Source: CAD feature listing. Evaluate the final solid. Frame: model axes, mm. A direction names the side the tool comes from. Coordinates: 2 decimals unless noted, no trailing zeros. Order: outer loops, then holes, each group sorted by start corner. A loop starts at its lowest first (then second) coordinate and runs counter-clockwise, first axis right, second up. Notation, with made-up numbers: (-25.75, -17) -> (24.25, -17) arc R23 ccw to (24.25, 0) -> close; hole circle Ø11 at (-21, 86.25). An arc over 180 degrees is marked (long way). Write each question's results on one line, items separated by ' | '. Start each with the question number.
Autodesk Inventor part; units mm, degrees
ref_plane "WorkPlane1" through (0, 0, 0) normal (0, 0, 1) x (1, 0, 0)
ref_plane "MSC_PF1" through (0, 0, 0) normal (1, 0, 0) x (0, 1, 0)
ref_plane "MSC_PT1" through (0, 0, 0) normal (0, 0, -1) x (-1, 0, 0)
ref_plane "WorkPlane1" through (0, 0, 0) normal (0, 0, 1) x (1, 0, 0)
sketch "Sketch1" plane through (0, 0, 0) normal (0, 0, 1) x (1, 0, 0)
  point P0 (0, 0)
sketch "Sketch2" plane through (0, 0, 0) normal (0, 0, 1) x (1, 0, 0)
  line L0 (-6.5, 3.7529) -> (-6.5, -3.7529)
  line L1 (0, 7.5054) -> (-6.5, 3.7529)
  line L2 (6.5, 3.7529) -> (0, 7.5054)
  line L3 (6.5, -3.7529) -> (6.5, 3.7529)
  line L4 (0, -7.5054) -> (6.5, -3.7529)
  line L5 (-6.5, -3.7529) -> (0, -7.5054)
  circle A0 centre (0, 0) radius 6.5 construction
  dimension "d1" = 13
  dimension "d29" = 0
  dimension "d30" = 0
extrude "Extrusion1" add sketch "Sketch2" along normal blind 5.3
sketch "Sketch3" plane through (0, 0, 0) normal (1, 0, 0) x (0, 1, 0)
  line L0 (6.5, 5.3) -> (7.6054, 5.3)
  line L1 (7.6054, 4.6618) -> (6.5, 5.3)
  line L2 (7.6054, 5.3) -> (7.6054, 4.6618)
  line L3 (0, -1.06) -> (0, 6.36)
  line L4 (7.5054, 0) -> (7.5054, 5.3)
  dimension "d25" = 0.1
  dimension "d26" = 0
  dimension "d27" = 60
  dimension "d28" = 6.5
revolve "Revolution1" cut sketch "Sketch3" angle 360 about axis through (0, 0, -10) along (0, 0, 1)
sketch "Sketch4" plane through (0, 0, 0) normal (1, 0, 0) x (0, 1, 0)
  line L0 (0, -30) -> (0, 0)
  line L1 (-4, -30) -> (0, -30)
  line L2 (-4, 0) -> (-4, -30)
  line L3 (0, 0) -> (-4, 0)
  line L4 (0, -30) -> (0, 0)
  line L5 (-4.8, 0) -> (0.8, 0)
  line L6 (0, -36) -> (0, 6)
  dimension "d18" = 4
  dimension "d20" = 30
  dimension "d33" = 0
  dimension "d34" = 0
revolve "Revolution2" add sketch "Sketch4" angle 360 about axis through (0, 0, -30) along (0, 0, -1)
chamfer "Chamfer1" distance 0.625 angle 45 1 edges at (0, 4, -30)
fillet "Fillet1" radius 0.4 1 edges at (0, 4, 0)
thread "Thread1"
ref_plane "MSC_PF1" through (0, 0, 0) normal (1, 0, 0) x (0, 1, 0)
ref_plane "MSC_PT1" through (0, 0, 0) normal (0, 0, -1) x (-1, 0, 0)
equation "\"d22\" = 0.5 * PTC"
equation "\"d23\" = 0.5 * PTC"
equation "\"d24\" = r"
equation "\"d1\" = ParS"
equation "\"d6\" = ParK"
equation "\"b\" = NLG - 2 * PTC"
equation "\"d28\" = 0.5 * ParS"
equation "\"d18\" = 0.5 * NND"
equation "\"d20\" = NLG"
equation "\"NND\" = 8"
equation "\"NLG\" = 30"
equation "\"PTC\" = 1.25"
equation "\"ParK\" = 5.3"
equation "\"ParS\" = 13"
equation "\"msp_es\" = 0.577367 * ParS"
equation "\"r\" = 0.4"
equation "\"THREADDIA\" = NND"
properties part number "ISO 4018 - M8 x 30" material "Steel"
(1) First-contact query: P1, Ø3, axis at y = 1.5, z = -9.5, coming from the +X side; P2, Ø2, axis at x = -0.5, z = -23.5, coming from the +Y side; P3, Ø2, axis at y = -4.5, z = -11, coming from the -X side. Flat tips, straight axial feed; report the tip coordinate or a pass-through.
(2) Section A-A on z = -15. Return the cut outline in (x, y).
(3) Line query: L1, parallel to Z at x = 2.5, y = -5.5; L2, parallel to Y at x = -3.25, z = 2; L3, parallel to Y at x = 5.5, z = 2.5. Output: solid intervals per line, ascending.
(4) Reachability of faces 1 (the flat face through (-4.4, -1.6, 0)), 2 (the flat face through (-3.2, 5.66, 2.61)) from +Z, -Z, +X, -X, +Y, -Y: full face, straight path, thin tool, end or side. Return the list, or none.
Results list:
1) P1: stops at x = 4 | P2: stops at y = 4 | P3: stops at x = -1.94
2) outline: circle Ø8 at (0, 0)
3) L1: z = 0 to 5.3 | L2: y = -5.63 to 5.63 | L3: y = -4.33 to 4.33
4) face 1: -Z | face 2: +Z, -Z, -X, +Y
